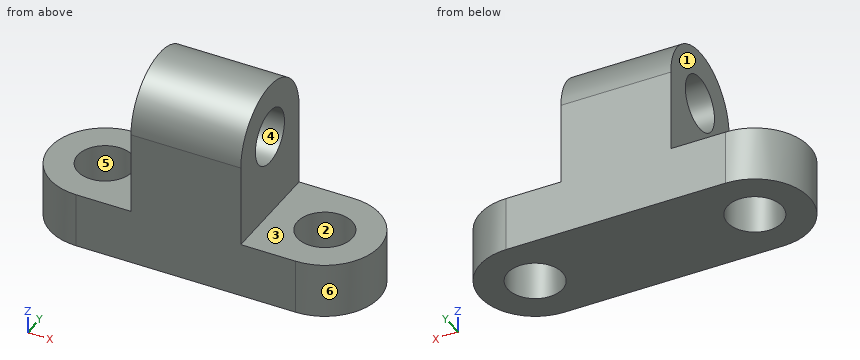
```python
from build123d import *

# Parameters (mm, degrees)
F1_DEPTH  = 25.4
F3_DEPTH  = 12.7
F5_DEPTH  = 12.7
F7_DEPTH  = 25.4
F8_R      = 6.352316
F9_DEPTH  = 25.4
F10_R     = 6.352482
F12_DEPTH = 25.4
F11_R     = 6.35
F13_DEPTH = 25.4


with BuildPart() as f1:
    # F0 (on Front) → F1 (new body)
    with BuildSketch(Plane.XZ):
        Polygon((-37.59941, 3.532893), (-37.59941, -9.167107), (13.20059, -9.167107), (13.20059, 3.532893), (0.50059, 3.532893), (0.50059, 22.582893), (-24.89941, 22.582893), (-24.89941, 3.532893), align=None)
    extrude(amount=F1_DEPTH)

    # F2 (on face) → F3 (join)
    with BuildSketch(Plane.XY.offset(3.532893)):
        with BuildLine():
            Line((13.20059, 0), (13.20059, -25.4))
            ThreePointArc((13.20059, -25.4), (25.90059, -12.7), (13.20059, 0))
        make_face()
    extrude(amount=-F3_DEPTH)

    # F4 (on face) → F5 (join)
    with BuildSketch(Plane.XY.offset(3.532893)):
        with BuildLine():
            Line((-37.59941, -25.4), (-37.59941, 0))
            ThreePointArc((-37.59941, 0), (-50.29941, -12.7), (-37.59941, -25.4))
        make_face()
    extrude(amount=-F5_DEPTH)

    # F6 (on face) → F7 (join)
    with BuildSketch(Plane(origin=(-24.89941, 0, 0), x_dir=(0, -1, 0), z_dir=(-1, 0, 0))):
        with BuildLine():
            Line((0, 22.582893), (25.4, 22.582893))
            ThreePointArc((25.4, 22.582893), (12.7, 35.282893), (0, 22.582893))
        make_face()
    extrude(amount=-F7_DEPTH)

    # F8 (on face) → F9 (cut)
    with BuildSketch(Plane(origin=(-24.89941, 0, 0), x_dir=(0, -1, 0), z_dir=(-1, 0, 0))):
        with Locations((12.7, 22.582893)):
            Circle(F8_R)
    extrude(amount=-F9_DEPTH, mode=Mode.SUBTRACT)

    # F10 (on face) → F12 (cut)
    with BuildSketch(Plane.XY.offset(3.532893)):
        with Locations((-37.59941, -12.7)):
            Circle(F10_R)
    extrude(amount=-F12_DEPTH, mode=Mode.SUBTRACT)

    # F11 (on face) → F13 (cut)
    with BuildSketch(Plane.XY.offset(3.532893)):
        with Locations((13.20059, -12.7)):
            Circle(F11_R)
    extrude(amount=-F13_DEPTH, mode=Mode.SUBTRACT)


solid = f1.part
```
The model under review builds one solid part; all positions refer to its coordinate system, in mm. Face numbers are marked on the shaded views. A direction names the side the tool comes from. Give positions to 0.01 mm unless a question says otherwise; leave off trailing zeros. Write each loop counter-clockwise with the first axis right and the second up, starting at its lowest first coordinate (ties: lowest second). Pieces come first, ordered by that corner, then holes. Notation, with made-up numbers: M -36,43 L -9,43 A32 cw -9,78 Z; hole C 5,16 d2. An arc over 180 degrees is marked long. Write each question's results on one line, items separated by ' | '. Start each with the question number.
1. Insertion check: pin 1 Ø5 at (y, z) = (-18, -3) entering from +X; pin 2 Ø3 at (y, z) = (-19, 2) entering from +X; pin 3 Ø12.5 at (x, y) = (-35.5, -14.5) entering from +Z. Each pin has a flat end and moves straight along its axis. Give the tip position at first contact, or say it passes through.
2. We need section C-C (x = 10). Write out the cut boundary in (y, z), and give its area (3 significant figures).
3. For probe 1 along X at (y, z) = (-12.75, -6.5); probe 2 along Z at (x, y) = (-19.5, -12.7); probe 3 along X at (y, z) = (-9, -1.5), list the stretches that pass through material, from the lowest coordinate up. Write a range as [from, to].
4. Mouldability with a two-part tool opening along X and no side actions: class the marked faces 4, 5 and 6 as released by +X, released by -X, zero draft, split by the parting line, or undercut.
5. We need section A-A (y = -12.7). Write out the cut boundary in (x, z), and give its area (3 significant figures).
6. We need section D-D (x = -18). Write out the cut boundary in (y, z).
7. We need section B-B (z = -2.5). Write out the cut boundary in (x, y), and give its area (3 significant figures).
8. For the marked faces 1, 2 and 3, list the 3-axis set-ups (+Z, -Z, +X, -X, +Y, -Y) from which the entire face can be reached by the end or side of a thin tool; tool diameter is ignored.
Results found:
1) pin 1: stops at x = 25.59 | pin 2: stops at x = 24.96 | pin 3: stops at z = 3.53
2) outline: M -25.4,-9.17 L -18.18,-9.17 L -18.18,3.53 L -25.4,3.53 Z; M -7.22,-9.17 L 0,-9.17 L 0,3.53 L -7.22,3.53 Z | area: 183 mm^2
3) probe 1: x = [-50.3, -43.95], [-31.25, 6.85], [19.55, 25.9] | probe 2: z = [-9.17, 16.23], [28.94, 35.28] | probe 3: x = [-49.75, -42.76], [-32.44, 8.04], [18.36, 25.35]
4) face 4: zero draft | face 5: undercut | face 6: released by +X
5) outline: M -50.3,-9.17 L -43.95,-9.17 L -43.95,3.53 L -50.3,3.53 Z; M -31.25,-9.17 L 6.85,-9.17 L 6.85,3.53 L 0.5,3.53 L 0.5,16.23 L -24.9,16.23 L -24.9,3.53 L -31.25,3.53 Z; M -24.9,28.94 L 0.5,28.94 L 0.5,35.28 L -24.9,35.28 Z; M 19.55,-9.17 L 25.9,-9.17 L 25.9,3.53 L 19.55,3.53 Z | area: 1,130 mm^2
6) outline: M -25.4,-9.17 L 0,-9.17 L 0,22.58 A12.7 ccw -25.4,22.58 Z; hole C -12.7,22.58 d12.7
7) outline: M -37.6,-25.4 L 13.2,-25.4 A12.7 ccw 13.2,0 L -37.6,0 A12.7 ccw Z; hole C -37.6,-12.7 d12.7; hole C 13.2,-12.7 d12.7 | area: 1,540 mm^2
8) face 1: +Z, -X, +Y, -Y | face 2: +Z, -Z | face 3: +Z, +X, +Y, -Y
